Drawing for the job (mm, zero at the part's lowest x, y, z). Give positions to 0.01 mm unless a question says otherwise; leave off trailing zeros. Write each loop counter-clockwise with the first axis right and the second up, starting at its lowest first coordinate (ties: lowest second). Pieces come first, ordered by that corner, then holes. Notation, with made-up numbers: M 74.5,-25 L 118.5,-25 A27 ccw 118.5,-9 Z; hole C 41.5,28 d8. An arc over 180 degrees is marked long. Answer as a JSON object with one key per item and string values. Group by question number.
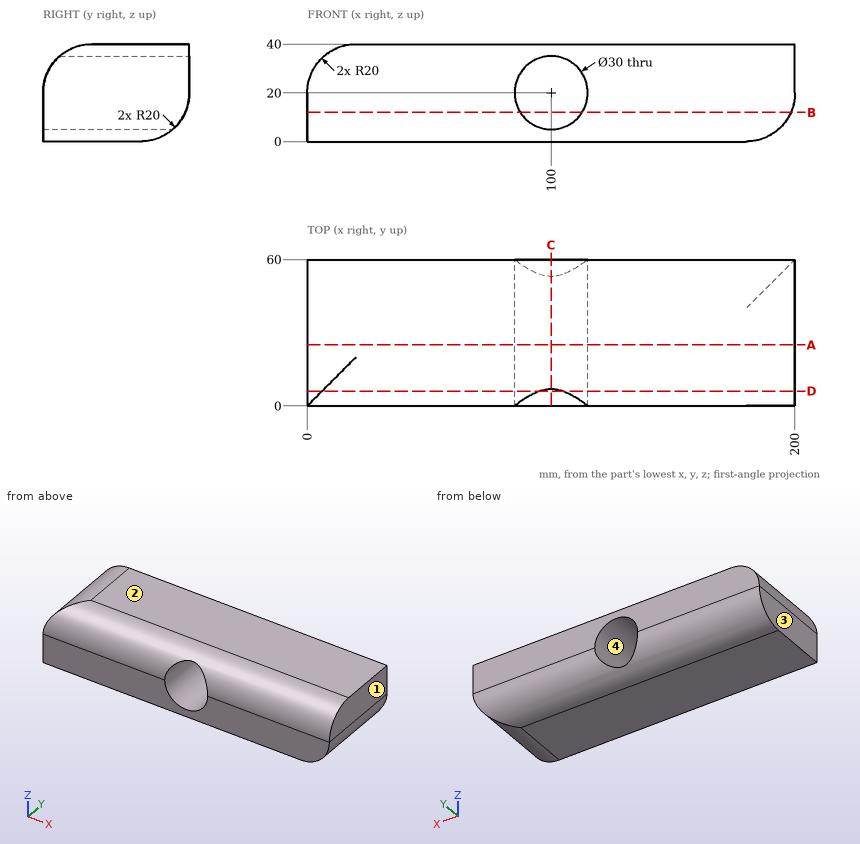
Q1. Slice it at D-D, the plane y = 6. Write the cut outline in (x, z), then the cut area to 3 significant figures.
Q2. Wall check: L1, parallel to Z at x = 100, y = 28.5; L2, parallel to Z at x = 93, y = 7; L3, parallel to X at y = 27.5, z = 23.5. Give the ranges that are in metal, low to high.
Q3. Slice it at C-C, the plane x = 100. Write the cut outline in (y, z), then the cut area to 3 significant figures.
Q4. Slice it at A-A, the plane y = 25. Write the cut outline in (x, z).
Q5. Drop flat-ended pins along their axis: P1, Ø2, axis at y = 43, z = 29, coming from the -X side; P2, Ø6, axis at x = 176.5, y = 6.5, coming from the +Z side; P3, Ø2, axis at x = 89.5, z = 14, coming from the +Y side; P4, Ø2, axis at x = 82, y = 17, coming from the +Z side. Give the stop position or say it passes through.
Q6. Slice it at B-B, the plane z = 12. Write the cut outline in (x, y).
Q7. Two-plate mould, pull along X, no slides. Class the marked faces 1, 2, 3 and 4: +X half, -X half, draft (parallel to the pull), parting line (faces both ways), or undercut.
Solved:
{
 "1": {"outline": "M 0,0 L 180,0 A20 ccw 200,20 L 200,34.28 L 104.58,34.28 A15 cw long 95.42,34.28 L 6,34.28 A20 ccw 0,20 Z", "area": "6,040 mm²"},
 "2": {"L1": "z = 0 to 5, 35 to 40", "L2": "z = 0 to 6.73, 33.27 to 35.2", "L3": "x = 0.31 to 85.41, 114.59 to 200"},
 "3": {"outline": "M 0,0 L 40,0 A20 ccw 53.23,5 L 0,5 Z; M 6.77,35 L 60,35 L 60,40 L 20,40 A20 ccw Z", "area": "491 mm²"},
 "4": {"outline": "M 0,0 L 180,0 A20 ccw 200,20 L 200,40 L 20,40 A20 ccw 0,20 Z; hole C 100,20 d30"},
 "5": {"P1": "stops at x = 1.67", "P2": "stops at z = 37.02", "P3": "passes through", "P4": "stops at z = 39.9"},
 "6": {"outline": "M 0,0 L 87.31,0 L 87.31,58.33 L 0,58.33 Z; M 112.69,0 L 198.33,0 L 198.33,58.33 L 112.69,58.33 Z"},
 "7": {"face 1": "+X half", "face 2": "draft", "face 3": "-X half", "face 4": "undercut"}
}
